from build123d import *

# Parameters (mm, degrees)
SKETCH1_R           = 1.5
BOSS_EXTRUDE1_DEPTH = 5


with BuildPart() as part:
    # Sketch1 → Boss-Extrude1 (new body)
    with BuildSketch(Plane(origin=(0, 0, 0), x_dir=(0, 0, -1), z_dir=(1, 0, 0))):
        with BuildLine():
            Line((44.162641246, 29.392068372), (44.162641246, 9.826128546))
            ThreePointArc((44.162641246, 9.826128546), (48.162641246, 5.826128546), (52.162641246, 9.826128546))
            Line((52.162641246, 9.826128546), (52.162641246, 29.392068372))
            ThreePointArc((52.162641246, 29.392068372), (51.137514981, 31.866942106), (48.662641246, 32.892068372))
            Line((48.662641246, 32.892068372), (47.662641246, 32.892068372))
            ThreePointArc((47.662641246, 32.892068372), (45.187767512, 31.866942106), (44.162641246, 29.392068372))
        make_face()
        with Locations((48.162641246, 30.051539634)):
            Circle(SKETCH1_R, mode=Mode.SUBTRACT)
        with Locations((48.162641246, 9.826128546)):
            Circle(SKETCH1_R, mode=Mode.SUBTRACT)
    extrude(amount=BOSS_EXTRUDE1_DEPTH)


solid = part.part
Source: CAD feature listing. Evaluate the final solid. Frame: model axes, mm. Round coordinates to 2 decimals unless told otherwise and drop trailing zeros. Loops run counter-clockwise (first coordinate to the right, second up) from the corner with the lowest first, then second, coordinate; pieces in that order, holes last. Notation, with made-up numbers: (37.25, 77.25) -> (42.25, 77.25) arc R21 ccw to (42.25, 89.25) -> close; hole circle Ø3 at (-38.75, 79.25). An arc over 180 degrees is marked (long way). Answer as a JSON object with one key per item and string values. Group by question number.
Q1. Section query C-C (z = -45). Output: boundary loops of the cut face in (x, y).
Q2. Ray query, line 1 (Y direction, x = 0.55, z = -47.5); line 2 (Y direction, x = 4.05, z = -47.25); line 3 (Z direction, x = 2.65, y = 9.5). Return the intervals inside material, ascending. Write a range as from..to.
Q3. Mould query, pull axis Y, two halves, no side actions, for faces 1 (the cylindrical face through (2.465, 5.827, -48.075)), 2 (the cylindrical face through (2.465, 8.913, -46.972)), 3 (the flat face through (2, 32.892, -48)). Classes: pulls with the +Y half, pulls with the -Y half, needs draft (parallel to the pull), parting line crosses it, or undercut.
Q4. Section query A-A (x = 1.8). Output: boundary loops of the cut face in (y, z), plus the area to 3 significant figures.
Q5. Section query B-B (z = -51). Output: boundary loops of the cut face in (x, y), plus the area to 3 significant figures.
Q6. Contact query for a flat-ended pin moving along its axis: P1, Ø2.5, axis at y = 30.05, z = -48.16, coming from the +X side. Output: stop coordinate, or through.
Completed:
{
 "1": {"outline": "(0, 7.38) -> (5, 7.38) -> (5, 31.66) -> (0, 31.66) -> close"},
 "2": {"line 1": "5.88..8.48, 11.17..28.71, 31.4..32.89", "line 2": "5.93..8.64, 11.02..28.86, 31.24..32.87", "line 3": "-52.15..-49.63, -46.7..-44.18"},
 "3": {"face 1": "pulls with the -Y half", "face 2": "undercut", "face 3": "pulls with the +Y half"},
 "4": {"outline": "(9.83, -52.16) -> (29.39, -52.16) arc R3.5 ccw to (32.89, -48.66) -> (32.89, -47.66) arc R3.5 ccw to (29.39, -44.16) -> (9.83, -44.16) arc R4 ccw to start; hole circle Ø3 at (9.83, -48.16); hole circle Ø3 at (30.05, -48.16)", "area": "190 mm²"},
 "5": {"outline": "(0, 7.01) -> (5, 7.01) -> (5, 32) -> (0, 32) -> close", "area": "125 mm²"},
 "6": {"P1": "through"}
}
